Work out the finished part from the listing and answer in its coordinate system (mm). Face numbers are marked on the shaded views. A direction names the side the tool comes from. Round coordinates to 2 decimals unless told otherwise and drop trailing zeros. Loops run counter-clockwise (first coordinate to the right, second up) from the corner with the lowest first, then second, coordinate; pieces in that order, holes last. Notation, with made-up numbers: (67.25, -13) -> (88.25, -13) arc R25 cw to (88.25, 19) -> close; hole circle Ø2 at (36.5, -39). An arc over 180 degrees is marked (long way). Use one line per item in the form item = value.
```python
from build123d import *

# Parameters (mm, degrees)
F1_DEPTH = 19.05
F2_R     = 3.175
F3_DEPTH = 25
F4_R     = 3.175
F5_DEPTH = 25


with BuildPart() as f1:
    # F0 (on Front) → F1 (new body)
    with BuildSketch(Plane.XZ):
        Polygon((0, 1.5875), (0, 0), (50, 0), (99.2403876506, 8.6824088833), (98.9647211686, 10.2457911913), (49.8611117467, 1.5875), align=None)
    extrude(amount=F1_DEPTH)

    # F2 (on face) → F3 (cut)
    with BuildSketch(Plane(origin=(0, 0, 0), x_dir=(1, 0, 0), z_dir=(0, 0, -1))):
        with Locations((25, 9.525)):
            Circle(F2_R)
    extrude(amount=-F3_DEPTH, mode=Mode.SUBTRACT)

    # F4 (on face) → F5 (cut)
    with BuildSketch(Plane(origin=(1.5076844804, 0, -8.5505035831), x_dir=(0.984807753, 0, 0.1736481777), z_dir=(0.1736481777, 0, -0.984807753))):
        with Locations((74.2403876506, 9.525)):
            Circle(F4_R)
    extrude(amount=-F5_DEPTH, mode=Mode.SUBTRACT)


solid = f1.part
```
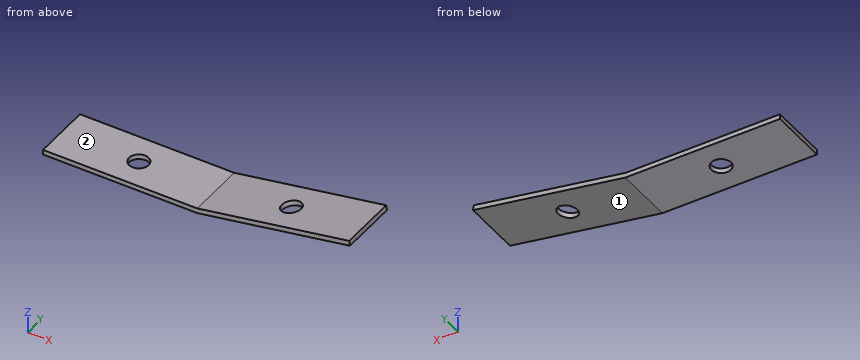
(1) Consider L1, parallel to Y at x = 25, z = 1.15; L2, parallel to Z at x = 31.5, y = -8.5; L3, parallel to Z at x = 57, y = -6.5. Determine where each line is inside the solid, lowest interval first.
Completed:
L1 = -19.05 to -12.7, -6.35 to 0
L2 = 0 to 1.59
L3 = 1.23 to 2.85
(2) Given P1, Ø5.5, axis at x = 12.5, y = -12, coming from the +Z side; P2, Ø4, axis at x = 78.5, y = -2.5, coming from the -Z side, each flat-ended and moving along its own axis, determine where each tip first touches the part or whether it passes through.
Completed:
P1 = 1.59
P2 = 4.67
(3) Find section D-D, the plane z = 2.75. Write down the section's boundary in (x, y).
Completed:
outline = (56.45, -19.05) -> (65.6, -19.05) -> (65.6, 0) -> (56.45, 0) -> close
(4) Find section B-B, the plane y = -11. Write down the section's boundary in (x, z), then the cut area to 3 significant figures.
Completed:
outline = (0, 0) -> (22.19, 0) -> (22.19, 1.59) -> (0, 1.59) -> close; (27.81, 0) -> (50, 0) -> (71.85, 3.85) -> (71.58, 5.42) -> (49.86, 1.59) -> (27.81, 1.59) -> close; (77.11, 6.39) -> (77.39, 4.83) -> (99.24, 8.68) -> (98.96, 10.25) -> close
area = 141 mm2
(5) Find section A-A, the plane x = 25. Write down the section's boundary in (y, z), then the cut area to 3 significant figures.
Completed:
outline = (-19.05, 0) -> (-12.7, 0) -> (-12.7, 1.59) -> (-19.05, 1.59) -> close; (-6.35, 0) -> (0, 0) -> (0, 1.59) -> (-6.35, 1.59) -> close
area = 20.2 mm2
(6) Find section C-C, the plane y = -15. Write down the section's boundary in (x, z).
Completed:
outline = (0, 0) -> (50, 0) -> (99.24, 8.68) -> (98.96, 10.25) -> (49.86, 1.59) -> (0, 1.59) -> close
(7) For the marked faces 1 and 2, determine the directions among +Z, -Z, +X, -X, +Y, -Y from which every point of the face is accessible in a straight line to the end or side of a thin tool.
Completed:
face_1 = -Z, +X, +Y, -Y
face_2 = +Z, -X, +Y, -Y
